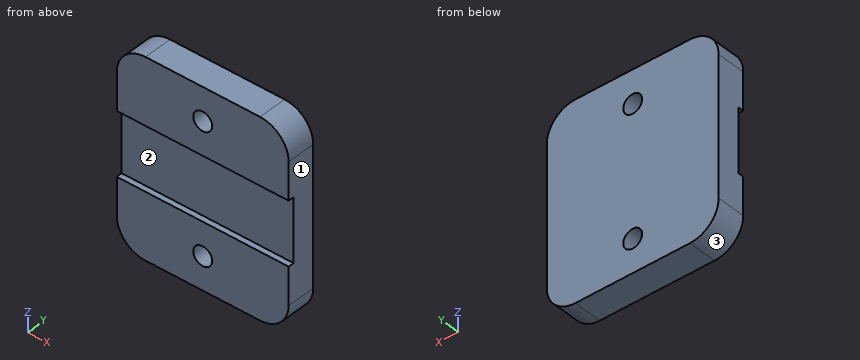
from build123d import *

# Parameters (mm, degrees)
SKETCH1_W           = 30
SKETCH1_H           = 34
BOSS_EXTRUDE1_DEPTH = 5
SKETCH2_W           = 11
SKETCH2_H           = 1
CUT_EXTRUDE1_DEPTH  = 31
FILLET1_R           = 5
SKETCH6_R           = 1.65
CUT_EXTRUDE2_DEPTH  = 6


with BuildPart() as part:
    # Sketch1 → Boss-Extrude1 (new body)
    with BuildSketch(Plane.XZ.offset(5)):
        Rectangle(SKETCH1_W, SKETCH1_H)
    extrude(amount=-BOSS_EXTRUDE1_DEPTH)

    # Sketch2 → Cut-Extrude1 (cut, through all)
    with BuildSketch(Plane.ZY.offset(15)):
        with Locations((0, -4.5)):
            Rectangle(SKETCH2_W, SKETCH2_H)
    extrude(amount=-CUT_EXTRUDE1_DEPTH, mode=Mode.SUBTRACT)

    # Fillet1
    fillet1_edges = [part.edges().sort_by_distance(p)[0] for p in [
        (15, -2.5, 17),
        (15, -2.5, -17),
        (-15, -2.5, -17),
        (-15, -2.5, 17),
    ]]
    fillet(fillet1_edges, radius=FILLET1_R)

    # Sketch6 → Cut-Extrude2 (cut, through all)
    with BuildSketch(Plane.XZ.offset(5)):
        with Locations((0, 11.25)):
            Circle(SKETCH6_R)
        with Locations((0, -11.25)):
            Circle(SKETCH6_R)
    extrude(amount=-CUT_EXTRUDE2_DEPTH, mode=Mode.SUBTRACT)


solid = part.part
For this review, take the finished solid that the model builds, in its own axes (mm). Face numbers are marked on the shaded views. Coordinates: 2 decimals unless noted, no trailing zeros. Order: outer loops, then holes, each group sorted by start corner. A loop starts at its lowest first (then second) coordinate and runs counter-clockwise, first axis right, second up. Notation, with made-up numbers: (45, 62) -> (80, 62) arc R28 cw to (80, 95) -> close; hole circle Ø3 at (-31, -30). An arc over 180 degrees is marked (long way). Return JSON: item names as keys, results as strings.
1. The part is to be moulded in two halves that separate along Z. For the marked faces 1, 2 and 3, say which applies: +Z half, -Z half, draft (parallel to the pull), parting line (faces both ways), or undercut.
Answer block:
{"face 1": "draft", "face 2": "undercut", "face 3": "-Z half"}
2. We need section D-D on y = -1.7. Write out the cut boundary in (x, z).
Answer block:
{"outline": "(-15, -12) arc R5 ccw to (-10, -17) -> (10, -17) arc R5 ccw to (15, -12) -> (15, 12) arc R5 ccw to (10, 17) -> (-10, 17) arc R5 ccw to (-15, 12) -> close; hole circle Ø3.3 at (0, -11.25); hole circle Ø3.3 at (0, 11.25)"}
3. For line 1 (Z direction, x = 0, y = -1.05); line 2 (Y direction, x = -8.75, z = -4); line 3 (Z direction, x = 10.25, y = -1.8), list the stretches that pass through material, from the lowest coordinate up. Write a range as from..to.
Answer block:
{"line 1": "-17..-12.9, -9.6..9.6, 12.9..17", "line 2": "-4..0", "line 3": "-16.99..16.99"}
4. For pin 1 Ø5.5 at (x, z) = (3, 1.5) entering from -Y, flat-tipped, find the tip position at first contact; note if it passes through.
Answer block:
{"pin 1": "y = -4"}
5. We need section B-B on z = 11.25. Write out the cut boundary in (x, y), and give its area (4 significant figures).
Answer block:
{"outline": "(-15, -5) -> (-1.65, -5) -> (-1.65, 0) -> (-15, 0) -> close; (1.65, -5) -> (15, -5) -> (15, 0) -> (1.65, 0) -> close", "area": "133.5 mm²"}
6. We need section C-C on x = 0. Write out the cut boundary in (y, z).
Answer block:
{"outline": "(-5, -17) -> (0, -17) -> (0, -12.9) -> (-5, -12.9) -> close; (-5, -9.6) -> (0, -9.6) -> (0, 9.6) -> (-5, 9.6) -> (-5, 5.5) -> (-4, 5.5) -> (-4, -5.5) -> (-5, -5.5) -> close; (-5, 12.9) -> (0, 12.9) -> (0, 17) -> (-5, 17) -> close"}
7. We need section A-A on y = -4.4. Write out the cut boundary in (x, z), and give its area (3 significant figures).
Answer block:
{"outline": "(-15, -12) arc R5 ccw to (-10, -17) -> (10, -17) arc R5 ccw to (15, -12) -> (15, -5.5) -> (-15, -5.5) -> close; (-15, 5.5) -> (15, 5.5) -> (15, 12) arc R5 ccw to (10, 17) -> (-10, 17) arc R5 ccw to (-15, 12) -> close; hole circle Ø3.3 at (0, -11.25); hole circle Ø3.3 at (0, 11.25)", "area": "651 mm²"}
